Geometry check sheet. Reference: the model listing, model coordinates, mm. Face numbers are marked on the shaded views. A direction names the side the tool comes from. Coordinates: 2 decimals unless noted, no trailing zeros. Write each loop counter-clockwise with the first axis right and the second up, starting at its lowest first coordinate (ties: lowest second). Pieces come first, ordered by that corner, then holes. Notation, with made-up numbers: M 29.5,-8.5 L 53.5,-8.5 A22 cw 53.5,1.5 Z; hole C 15,-28.5 d10. An arc over 180 degrees is marked long. Answer as a JSON object with one key per item and string values. Group by question number.
```python
from build123d import *

# Parameters (mm, degrees)
SKETCH1_W           = 19
SKETCH1_H           = 16
BOSS_EXTRUDE1_DEPTH = 11
SHELL1_T            = -2
SKETCH2_R           = 0.625
CUT_EXTRUDE1_DEPTH  = 10


with BuildPart() as part:
    # Sketch1 → Boss-Extrude1 (new body)
    with BuildSketch(Plane(origin=(0, 0, 0), x_dir=(1, 0, 0), z_dir=(0, 1, 0))):
        with Locations((9.5, 8)):
            Rectangle(SKETCH1_W, SKETCH1_H)
    extrude(amount=BOSS_EXTRUDE1_DEPTH)

    # Shell1
    shell1_openings = [part.faces().sort_by_distance(p)[0] for p in [
        (9.5, 11, -8),
    ]]
    offset(amount=SHELL1_T, openings=shell1_openings, kind=Kind.INTERSECTION)

    # Sketch2 → Cut-Extrude1 (cut)
    with BuildSketch(Plane(origin=(0, 2, 0), x_dir=(1, 0, 0), z_dir=(0, 1, 0))):
        with Locations((16.025684832, 11.778007382)):
            Circle(SKETCH2_R)
        with Locations((16.025684832, 6.698007382)):
            Circle(SKETCH2_R)
        with Locations((16.025684832, 4.158007382)):
            Circle(SKETCH2_R)
    extrude(amount=-CUT_EXTRUDE1_DEPTH, mode=Mode.SUBTRACT)


solid = part.part
```
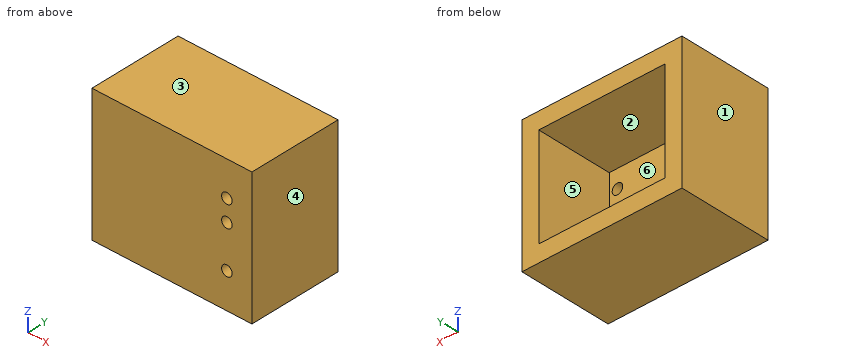
1) Draft check along Z on the marked faces 3, 4, 5 and 6. Enter one of: +Z half, -Z half, draft (parallel to the pull), parting line (faces both ways), or undercut.
2) Section check A-A (y = 5.75). Record the cut outline in (x, z).
3) Section check D-D (z = -8.5). Record the cut outline in (x, y).
4) Go/stop test with flat-tipped pins: pin 1 Ø1.1 at (x, z) = (16.03, -11.78) entering from -Y; pin 2 Ø9.5 at (x, z) = (10.5, -9) entering from +Y. Record where each tip stops, or that it passes through.
5) Section check C-C (z = -11.5). Record the cut outline in (x, y), then the cut area to 3 significant figures.
6) Section check B-B (x = 3.5). Record the cut outline in (y, z), then the cut area to 3 significant figures.
7) Set-up check for the marked faces 1 and 2: record each of +Z, -Z, +X, -X, +Y, -Y from which the full face is reachable in a straight line by a thin tool's end or side.
8) Material ranges on probe 1 along Z at (x, y) = (5.5, 3); probe 2 along X at (y, z) = (5.5, -7.25); probe 3 along Y at (x, z) = (11.75, -9.25), recorded low to high. Write a range as [from, to].
Entries:
{
 "1": {"face 3": "+Z half", "face 4": "draft", "face 5": "undercut", "face 6": "undercut"},
 "2": {"outline": "M 0,-16 L 19,-16 L 19,0 L 0,0 Z; hole M 2,-14 L 17,-14 L 17,-2 L 2,-2 Z"},
 "3": {"outline": "M 0,0 L 19,0 L 19,11 L 17,11 L 17,2 L 2,2 L 2,11 L 0,11 Z"},
 "4": {"pin 1": "through", "pin 2": "y = 2"},
 "5": {"outline": "M 0,0 L 15.47,0 L 15.47,2 L 2,2 L 2,11 L 0,11 Z; M 16.59,0 L 19,0 L 19,11 L 17,11 L 17,2 L 16.59,2 Z", "area": "71.8 mm^2"},
 "6": {"outline": "M 0,-16 L 11,-16 L 11,-14 L 2,-14 L 2,-2 L 11,-2 L 11,0 L 0,0 Z", "area": "68.0 mm^2"},
 "7": {"face 1": "+Z, -Z, -X, +Y, -Y", "face 2": "+Y"},
 "8": {"probe 1": "[-16, -14], [-2, 0]", "probe 2": "[0, 2], [17, 19]", "probe 3": "[0, 2]"}
}
